from build123d import *

# Parameters (mm, degrees)
MAIN_PROFILE_SKETCH_W       = 110
MAIN_PROFILE_SKETCH_H       = 37
MAIN_EXTRUSION_DEPTH        = 10
DETAIL_PROFILE_2_SKETCH_R   = 3
DETAIL_EXTRUSION_2_DEPTH    = 1.5
DETAIL_PROFILE_3_SKETCH_R   = 3
DETAIL_PROFILE_3_SKETCH_W   = 21.8
DETAIL_PROFILE_3_SKETCH_H   = 41
DETAIL_PROFILE_3_SKETCH_W_2 = 49.6
DETAIL_EXTRUSION_3_DEPTH    = 0.2
DETAIL_PROFILE_4_SKETCH_R   = 1.7
DETAIL_PROFILE_4_SKETCH_W   = 49.6
DETAIL_PROFILE_4_SKETCH_H   = 41
DETAIL_PROFILE_4_SKETCH_W_2 = 21.8
DETAIL_EXTRUSION_4_DEPTH    = 1.3


with BuildPart() as part:
    # Main Profile Sketch → Main Extrusion (new body)
    with BuildSketch(Plane.XY.offset(61.5)):
        with BuildLine():
            Line((-272, -6), (-158, -6))
            Line((-158, -6), (-158, -47))
            Line((-158, -47), (-265.887822961, -47))
            ThreePointArc((-265.887822961, -47), (-268.700050917, -45.258804298), (-272, -45.484025518))
            Line((-272, -45.484025518), (-272, -6))
        make_face()
        with Locations((-215, -26.5)):
            Rectangle(MAIN_PROFILE_SKETCH_W, MAIN_PROFILE_SKETCH_H, mode=Mode.SUBTRACT)
    extrude(amount=-MAIN_EXTRUSION_DEPTH)

    # Detail Profile 2 Sketch → Detail Extrusion 2 (add)
    with BuildSketch(Plane.XY.offset(51.5)):
        with BuildLine():
            Line((-272, -6), (-158, -6))
            Line((-158, -6), (-158, -47))
            Line((-158, -47), (-265.887822961, -47))
            ThreePointArc((-265.887822961, -47), (-268.700050917, -45.258804298), (-272, -45.484025518))
            Line((-272, -45.484025518), (-272, -6))
        make_face()
        with Locations((-263, -26.5)):
            Circle(DETAIL_PROFILE_2_SKETCH_R, mode=Mode.SUBTRACT)
        with Locations((-167, -26.5)):
            Circle(DETAIL_PROFILE_2_SKETCH_R, mode=Mode.SUBTRACT)
    extrude(amount=-DETAIL_EXTRUSION_2_DEPTH)

    # Detail Profile 3 Sketch → Detail Extrusion 3 (add)
    # profile 1 of 3: a face of its own
    with BuildSketch(Plane.XY.offset(50)):
        with BuildLine():
            Line((-272, -6), (-250.2, -6))
            Line((-250.2, -6), (-250.2, -47))
            Line((-250.2, -47), (-265.887822961, -47))
            ThreePointArc((-265.887822961, -47), (-268.700050917, -45.258804298), (-272, -45.484025518))
            Line((-272, -45.484025518), (-272, -6))
        make_face()
        with Locations((-263, -26.5)):
            Circle(DETAIL_PROFILE_3_SKETCH_R, mode=Mode.SUBTRACT)
    # profile 2 of 3: a face of its own
    with BuildSketch(Plane.XY.offset(50)):
        with Locations((-168.9, -26.5)):
            Rectangle(DETAIL_PROFILE_3_SKETCH_W, DETAIL_PROFILE_3_SKETCH_H)
        with Locations((-167, -26.5)):
            Circle(DETAIL_PROFILE_3_SKETCH_R, mode=Mode.SUBTRACT)
    # profile 3 of 3: a face of its own
    with BuildSketch(Plane.XY.offset(50)):
        with Locations((-215, -26.5)):
            Rectangle(DETAIL_PROFILE_3_SKETCH_W_2, DETAIL_PROFILE_3_SKETCH_H)
    extrude(amount=-DETAIL_EXTRUSION_3_DEPTH)

    # Detail Profile 4 Sketch → Detail Extrusion 4 (add)
    # profile 1 of 3: a face of its own
    with BuildSketch(Plane.XY.offset(49.8)):
        with BuildLine():
            Line((-272, -6), (-250.2, -6))
            Line((-250.2, -6), (-250.2, -47))
            Line((-250.2, -47), (-265.887822961, -47))
            ThreePointArc((-265.887822961, -47), (-268.700050917, -45.258804298), (-272, -45.484025518))
            Line((-272, -45.484025518), (-272, -6))
        make_face()
        with Locations((-263, -26.5)):
            Circle(DETAIL_PROFILE_4_SKETCH_R, mode=Mode.SUBTRACT)
    # profile 2 of 3: a face of its own
    with BuildSketch(Plane.XY.offset(49.8)):
        with Locations((-215, -26.5)):
            Rectangle(DETAIL_PROFILE_4_SKETCH_W, DETAIL_PROFILE_4_SKETCH_H)
    # profile 3 of 3: a face of its own
    with BuildSketch(Plane.XY.offset(49.8)):
        with Locations((-168.9, -26.5)):
            Rectangle(DETAIL_PROFILE_4_SKETCH_W_2, DETAIL_PROFILE_4_SKETCH_H)
        with Locations((-167, -26.5)):
            Circle(DETAIL_PROFILE_4_SKETCH_R, mode=Mode.SUBTRACT)
    extrude(amount=-DETAIL_EXTRUSION_4_DEPTH)


solid = part.part
Geometry: final body of the model. Coordinates: model frame, mm. A direction names the side the tool comes from. Round coordinates to 2 decimals unless told otherwise and drop trailing zeros. Loops run counter-clockwise (first coordinate to the right, second up) from the corner with the lowest first, then second, coordinate; pieces in that order, holes last. Notation, with made-up numbers: (48, -38) -> (61, -38) arc R25 cw to (61, -11) -> close; hole circle Ø3 at (-38, 87.5). An arc over 180 degrees is marked (long way). One line per question, with ' | ' between items. Start each with the question number.
1. Set-up query: faces 1 (the face through (-165.38, -25.99, 49.16)), 2 (the face through (-216, -8, 57)), 3 (the face through (-245, -26, 50)). Return all of +Z, -Z, +X, -X, +Y, -Y with unobstructed straight access to the full face (end or side cutting, diameter ignored); none if empty.
2. Line query: line 1 along Y through (x, z) = (-263, 50.7); line 2 along Y through (x, z) = (-167, 49.1); line 3 along X through (y, z) = (-10.5, 53). Output: solid intervals per line, ascending. Write a range as [from, to].
3. Section C-C on y = -26.5. Count the separate pieces of the cut face and the enclosed holes in it, and give its area (3 significant figures).
4. Contact query for flat-ended pins moving along their axis: pin 1 (3 mm diameter, centred on x = -261.5, y = -27, fed in from +Z); pin 2 (4 mm diameter, centred on x = -185, y = -16, fed in from -Z); pin 3 (3 mm diameter, centred on x = -263, y = -26.5, fed in from -Z); pin 4 (4 mm diameter, centred on x = -167, y = -26.5, fed in from +Z). Output: stop coordinate, or through.
5. Section A-A on x = -263. Output: boundary loops of the cut face in (y, z), and give its area (3 significant figures).
6. Mould query, pull axis Y, two halves, no side actions, for faces 4 (the face through (-268.65, -45.27, 55.09)), 5 (the face through (-261, -26, 48.5)), 6 (the face through (-270, -27, 57)). Classes: pulls with the +Y half, pulls with the -Y half, needs draft (parallel to the pull), parting line crosses it, or undercut.
7. Section B-B on z = 58.75. Output: boundary loops of the cut face in (x, y).
8. Section D-D on y = -13.5. Output: boundary loops of the cut face in (x, z), and give its area (3 significant figures).
Returned:
1) face 1: +Z, -Z | face 2: +Z | face 3: -Z, +Y, -Y
2) line 1: y = [-47, -29.5], [-23.5, -6] | line 2: y = [-47, -28.2], [-24.8, -6] | line 3: x = [-272, -270], [-160, -158]
3) separate pieces: 3 | enclosed holes: 0 | area: 322 mm2
4) pin 1: stops at z = 51.5 | pin 2: stops at z = 50 | pin 3: passes through | pin 4: stops at z = 49.8
5) outline: (-47, 48.5) -> (-28.2, 48.5) -> (-28.2, 49.8) -> (-29.5, 49.8) -> (-29.5, 51.5) -> (-45, 51.5) -> (-45, 61.5) -> (-47, 61.5) -> close; (-24.8, 48.5) -> (-6, 48.5) -> (-6, 61.5) -> (-8, 61.5) -> (-8, 51.5) -> (-23.5, 51.5) -> (-23.5, 49.8) -> (-24.8, 49.8) -> close | area: 148 mm2
6) face 4: pulls with the -Y half | face 5: needs draft | face 6: undercut
7) outline: (-272, -45.48) arc R5.4 cw to (-265.89, -47) -> (-158, -47) -> (-158, -6) -> (-272, -6) -> close; hole (-270, -45) -> (-160, -45) -> (-160, -8) -> (-270, -8) -> close
8) outline: (-272, 48.5) -> (-250.2, 48.5) -> (-250.2, 50) -> (-239.8, 50) -> (-239.8, 48.5) -> (-190.2, 48.5) -> (-190.2, 50) -> (-179.8, 50) -> (-179.8, 48.5) -> (-158, 48.5) -> (-158, 61.5) -> (-160, 61.5) -> (-160, 51.5) -> (-270, 51.5) -> (-270, 61.5) -> (-272, 61.5) -> close | area: 351 mm2
